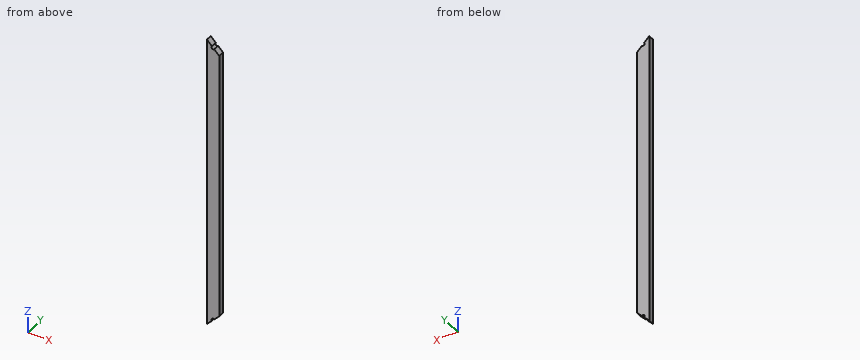
```python
from build123d import *

# Parameters (mm, degrees)
SKETCH1_W           = 14
SKETCH1_H           = 7
BOSS_EXTRUDE1_DEPTH = 330
CUT_EXTRUDE1_DEPTH  = 8
CUT_EXTRUDE2_DEPTH  = 8


with BuildPart() as part:
    # Sketch1 → Boss-Extrude1 (new body)
    with BuildSketch(Plane.XY):
        with Locations((7, 3.5)):
            Rectangle(SKETCH1_W, SKETCH1_H)
    extrude(amount=BOSS_EXTRUDE1_DEPTH)

    # Sketch2 → Cut-Extrude1 (cut, through all)
    with BuildSketch(Plane(origin=(0, 7, 0), x_dir=(1, 0, 0), z_dir=(0, 1, 0))):
        Polygon((0, 0), (14, -14), (14, 0), align=None)
        Polygon((14, -330), (0, -330), (14, -316), align=None)
    extrude(amount=-CUT_EXTRUDE1_DEPTH, mode=Mode.SUBTRACT)

    # Sketch3 → Cut-Extrude2 (cut, through all)
    with BuildSketch(Plane(origin=(0, 7, 0), x_dir=(1, 0, 0), z_dir=(0, 1, 0))):
        with BuildLine():
            Line((5.727207794, -5.727207794), (8.272792206, -8.272792206))
            ThreePointArc((8.272792206, -8.272792206), (5.727207794, -8.272792206), (5.727207794, -5.727207794))
        make_face()
        with BuildLine():
            Line((5.727207794, -324.272792206), (8.272792206, -321.727207794))
            ThreePointArc((8.272792206, -321.727207794), (5.727207794, -321.727207794), (5.727207794, -324.272792206))
        make_face()
    extrude(amount=-CUT_EXTRUDE2_DEPTH, mode=Mode.SUBTRACT)


solid = part.part
```
Read the model definition and answer for the solid it produces. Units are mm, in the model's axes. Give positions to 0.01 mm unless a question says otherwise; leave off trailing zeros. Loops run counter-clockwise (first coordinate to the right, second up) from the corner with the lowest first, then second, coordinate; pieces in that order, holes last.
Item 1: The part is cut by section B-B (x = 2.5). Write down the section's boundary in (y, z), and give its area (4 significant figures).
Item 2: Find the intervals of material crossed by line 1 along Z through (x, y) = (5.5, 4.75); line 2 along Z through (x, y) = (7.25, 1.5); line 3 along Z through (x, y) = (10, 0.5), in increasing order.
Item 3: The part is cut by section A-A (y = 5.75). Write down the section's boundary in (x, z).
Item 4: This flat-tipped pin is pushed along its axis until it touches: pin 1 Ø1 at (x, y) = (3, 4.5) entering from +Z. Where does it stop, or does it pass through?
Taken from the geometry:
1. outline: (0, 2.5) - (7, 2.5) - (7, 327.5) - (0, 327.5) - close
1. area: 2,275 mm2
2. line 1: z = 5.5 to 6.01, 7.99 to 322.01, 323.99 to 324.5
2. line 2: z = 8.78 to 321.22
2. line 3: z = 10 to 320
3. outline: (0, 0) - (5.73, 5.73) arc R1.8 cw to (8.27, 8.27) - (14, 14) - (14, 316) - (8.27, 321.73) arc R1.8 cw to (5.73, 324.27) - (0, 330) - close
4. pin 1: stops at z = 327.5
